Part model, mm, in its own coordinate system. A direction names the side the tool comes from. Coordinates: 2 decimals unless noted, no trailing zeros. Write each loop counter-clockwise with the first axis right and the second up, starting at its lowest first coordinate (ties: lowest second). Pieces come first, ordered by that corner, then holes. Notation, with made-up numbers: (73.5, 34.5) - (127.5, 34.5) arc R29 cw to (127.5, 63.5) - close; hole circle Ø1 at (48, 65.25). An arc over 180 degrees is marked (long way). Use a Markdown table: item, result.
```python
from build123d import *

# Parameters (mm, degrees)
EXTRUDE_1_DEPTH     = 2.4
SKETCH_2_W          = 6.85
SKETCH_2_H          = 1.4
EXTRUDE_2_DEPTH     = 7.65
SKETCH_3_W          = 6.85
SKETCH_3_H          = 1.4
EXTRUDE_3_DEPTH     = 1.2
SKETCH_5_W          = 6.85
SKETCH_5_H          = 1.4
SKETCH_6_W          = 1.2
SKETCH_6_H          = 2.5
EXTRUDE_4_DEPTH     = 2.8
CUT_EXTRUDE_1_DEPTH = 8.4
SKETCH_8_R          = 0.75
CUT_EXTRUDE_2_DEPTH = 22.65


with BuildPart() as part:
    # 草图1 → 凸台-拉伸1 (new body, symmetric)
    with BuildSketch(Plane.XY):
        Polygon((-22.75, 7.35), (-22.75, 0), (22.75, 0), (22.75, 7.35), (19.75, 7.35), (19.75, 18.65), (8.95, 18.65), (8.95, 7.35), align=None)
    extrude(amount=EXTRUDE_1_DEPTH, both=True)

    # 草图2 → 凸台-拉伸2 (add)
    with BuildSketch(Plane(origin=(0, 7.35, 0), x_dir=(1, 0, 0), z_dir=(0, 1, 0))):
        with Locations((-10.825, 0)):
            Rectangle(SKETCH_2_W, SKETCH_2_H)
        with Locations((-0.175, 0)):
            Rectangle(SKETCH_2_W, SKETCH_2_H)
    extrude(amount=EXTRUDE_2_DEPTH)

    # 草图3 → 凸台-拉伸3 (add)
    with BuildSketch(Plane(origin=(0, 15, 0), x_dir=(1, 0, 0), z_dir=(0, 1, 0))):
        with Locations((-0.175, 0)):
            Rectangle(SKETCH_3_W, SKETCH_3_H)
    extrude(amount=EXTRUDE_3_DEPTH)

    # 扫描1: sweep along a path in 草图4
    with BuildLine(Plane(origin=(0, 0, 0), x_dir=(0, 0, -1), z_dir=(1, 0, 0))) as sweep_1_path:
        Line((0, 0), (0, -1.3))
        ThreePointArc((0, -1.3), (0.292893219, -2.007106781), (1, -2.3))
        Line((1, -2.3), (5, -2.3))
    # 草图5 → 扫描1 (sweep)
    with BuildSketch(Plane.XZ):
        with Locations((-0.175, 0)):
            Rectangle(SKETCH_5_W, SKETCH_5_H)
        with Locations((-10.825, 0)):
            Rectangle(SKETCH_5_W, SKETCH_5_H)
    sweep(path=sweep_1_path.line)

    # 草图6 → 凸台-拉伸4 (add)
    with BuildSketch(Plane.XZ):
        with Locations((16.75, -1.15)):
            Rectangle(SKETCH_6_W, SKETCH_6_H)
        with Locations((19.15, -1.15)):
            Rectangle(SKETCH_6_W, SKETCH_6_H)
        with Locations((14.35, -1.15)):
            Rectangle(SKETCH_6_W, SKETCH_6_H)
        with Locations((11.95, -1.15)):
            Rectangle(SKETCH_6_W, SKETCH_6_H)
        with Locations((9.55, -1.15)):
            Rectangle(SKETCH_6_W, SKETCH_6_H)
    extrude(amount=EXTRUDE_4_DEPTH)

    # 草图7 → 切除-拉伸1 (cut, through all)
    with BuildSketch(Plane.XY.offset(2.4)):
        with BuildLine():
            Line((-21.584495188, 4.475), (-22.75, 4.475))
            Line((-22.75, 4.475), (-22.75, 2.875))
            Line((-22.75, 2.875), (-21.584495188, 2.875))
            ThreePointArc((-21.584495188, 2.875), (-18.225, 3.675), (-21.584495188, 4.475))
        make_face()
        with BuildLine():
            Line((22.75, 2.875), (22.75, 4.475))
            Line((22.75, 4.475), (21.584495188, 4.475))
            ThreePointArc((21.584495188, 4.475), (18.225, 3.675), (21.584495188, 2.875))
            Line((21.584495188, 2.875), (22.75, 2.875))
        make_face()
    extrude(amount=-CUT_EXTRUDE_1_DEPTH, mode=Mode.SUBTRACT)

    # 草图8 → 切除-拉伸2 (cut, through all)
    with BuildSketch(Plane(origin=(0, 18.65, 0), x_dir=(1, 0, 0), z_dir=(0, 1, 0))):
        with Locations((10.706638524, 0)):
            Circle(SKETCH_8_R)
        with Locations((13.135546175, 0)):
            Circle(SKETCH_8_R)
        with Locations((15.564453825, 0)):
            Circle(SKETCH_8_R)
        with Locations((17.993361476, 0)):
            Circle(SKETCH_8_R)
    extrude(amount=-CUT_EXTRUDE_2_DEPTH, mode=Mode.SUBTRACT)


solid = part.part
```
Item 1: Band-saw the part on C-C, the plane z = -4.25. Give the cut face in (x, y), then the cut area to 3 significant figures.
From the geometry:
| item | result |
|---|---|
| outline | (-14.25, -3) - (-7.4, -3) - (-7.4, -1.6) - (-14.25, -1.6) - close; (-3.6, -3) - (3.25, -3) - (3.25, -1.6) - (-3.6, -1.6) - close |
| area | 19.2 mm^2 |
Item 2: Drop flat-ended pins along their axis: P1, Ø4, axis at x = -16.5, z = -0.5, coming from the -Y side; P2, Ø3.5, axis at x = -9.5, y = 11, coming from the +Z side; P3, Ø1.3, axis at x = -22.5, z = 0, coming from the +Y side. Give the stop position or say it passes through.
From the geometry:
| item | result |
|---|---|
| P1 | y = 0 |
| P2 | z = 0.7 |
| P3 | y = 7.35 |
Item 3: Which spindle directions (+Z, -Z, +X, -X, +Y, -Y) get a long thin tool onto all of the face, cutting with end or side? Do faces 4 (the face through (17, -1, 0.1)), 5 (the face through (-11, -1, 0.7)), 6 (the face through (13.75, -1, -1)), 7 (the face through (17, -2.8, -1)), 8 (the face through (22, 2.875, 0)). Say none if no direction does.
From the geometry:
| item | result |
|---|---|
| face 4 | +Z, +X, -Y |
| face 5 | +Z, +X, -X, -Y |
| face 6 | +Z, -Z, -Y |
| face 7 | +Z, -Z, +X, -Y |
| face 8 | +Z, -Z, +X |
Item 4: Band-saw the part on A-A, the plane x = -20. Give the cut face in (y, z), then the cut area to 3 significant figures.
From the geometry:
| item | result |
|---|---|
| outline | (0, -2.4) - (1.9, -2.4) - (1.9, 2.4) - (0, 2.4) - close; (5.45, -2.4) - (7.35, -2.4) - (7.35, 2.4) - (5.45, 2.4) - close |
| area | 18.2 mm^2 |
Item 5: Two-plate mould, pull along X, no slides. Class faces 1 (the face through (17.35, -1, -1)), 2 (the face through (-11, -1, -0.7)), 3 (the face through (22.75, 1, 0)): pulls with the +X half, pulls with the -X half, needs draft (parallel to the pull), parting line crosses it, or undercut.
From the geometry:
| item | result |
|---|---|
| face 1 | undercut |
| face 2 | needs draft |
| face 3 | pulls with the +X half |
Item 6: Drill centre lines: probe 1 along X at (y, z) = (6.75, 0); probe 2 along Y at (x, z) = (-20, 1.25); probe 3 along Z at (x, y) = (11, 14.75). Where is each one in solid material? Low to high.
From the geometry:
| item | result |
|---|---|
| probe 1 | -22.75 to 9.96, 11.46 to 12.39, 13.89 to 14.81, 16.31 to 17.24, 18.74 to 22.75 |
| probe 2 | 0 to 1.9, 5.45 to 7.35 |
| probe 3 | -2.4 to -0.69, 0.69 to 2.4 |
Item 7: Band-saw the part on B-B, the plane y = 1.25. Give the cut face in (x, z).
From the geometry:
| item | result |
|---|---|
| outline | (-22.75, -2.4) - (22.75, -2.4) - (22.75, 2.4) - (-22.75, 2.4) - close; hole circle Ø1.5 at (10.71, 0); hole circle Ø1.5 at (13.14, 0); hole circle Ø1.5 at (15.56, 0); hole circle Ø1.5 at (17.99, 0) |
